```python
from build123d import *

# Parameters (mm, degrees)
BOSS_EXTRUDE1_DEPTH = 3.2
SKETCH3_R           = 12.3
BOSS_EXTRUDE2_DEPTH = 3.2
SKETCH4_R           = 4
BOSS_EXTRUDE3_DEPTH = 4
SKETCH6_W           = 3.2
SKETCH6_H           = 65
BOSS_EXTRUDE4_DEPTH = 190
SKETCH8_W           = 3.2
SKETCH8_H           = 89
BOSS_EXTRUDE5_DEPTH = 190
SKETCH9_W           = 194.2
SKETCH9_H           = 190
BOSS_EXTRUDE7_DEPTH = 3.2


with BuildPart() as part:
    # Sketch1 → Boss-Extrude1 (new body)
    with BuildSketch(Plane(origin=(0, 0, 0), x_dir=(1, 0, 0), z_dir=(0, 1, 0))):
        Polygon((-71.199297972, 0), (119.800702028, 0), (119.800702028, -90), (46.272924854, -150.155348756), (-15.035731115, -153.181069815), (-74.399297972, -109), (-74.399297972, -65), (-71.199297972, -65), align=None)
    boss_extrude1 = extrude(amount=BOSS_EXTRUDE1_DEPTH)

    # Sketch3 → Boss-Extrude2 (add)
    with BuildSketch(Plane.XZ):
        with Locations(Location((-5.399297972, 108.199281837, 0), (0, 0, 270))):
            Circle(SKETCH3_R)
    extrude(amount=BOSS_EXTRUDE2_DEPTH)

    # Sketch4 → Boss-Extrude3 (add)
    with BuildSketch(Plane.XZ.offset(3.2)):
        with Locations(Location((-5.399297972, 108.199281837, 0), (0, 0, 270))):
            Circle(SKETCH4_R)
    extrude(amount=BOSS_EXTRUDE3_DEPTH)

    # Sketch6 → Boss-Extrude4 (add)
    with BuildSketch(Plane(origin=(0, 0, 0), x_dir=(1, 0, 0), z_dir=(0, 1, 0))):
        with Locations((-72.799297972, -32.5)):
            Rectangle(SKETCH6_W, SKETCH6_H)
    extrude(amount=BOSS_EXTRUDE4_DEPTH)

    # Sketch8 → Boss-Extrude5 (add)
    with BuildSketch(Plane(origin=(0, 0, 0), x_dir=(1, 0, 0), z_dir=(0, 1, 0))):
        with Locations((118.200702028, -44.5)):
            Rectangle(SKETCH8_W, SKETCH8_H)
    extrude(amount=BOSS_EXTRUDE5_DEPTH)

    # Mirror1: Boss-Extrude1 across plane
    add(boss_extrude1.mirror(Plane(origin=(0, 95, 0), x_dir=(0, 0, 1), z_dir=(0, -1, 0))))

    # Sketch9 → Boss-Extrude7 (add)
    with BuildSketch(Plane.XY):
        with Locations((22.700702028, 95)):
            Rectangle(SKETCH9_W, SKETCH9_H)
    extrude(amount=-BOSS_EXTRUDE7_DEPTH)


solid = part.part
```
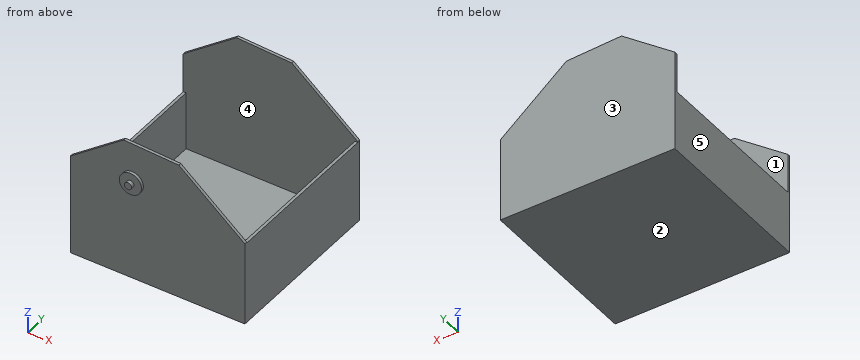
Design review of the part built by this model. Coordinates are the model's own, in mm. Face numbers are marked on the shaded views. A direction names the side the tool comes from. Give positions to 0.01 mm unless a question says otherwise; leave off trailing zeros. Write each loop counter-clockwise with the first axis right and the second up, starting at its lowest first coordinate (ties: lowest second). Pieces come first, ordered by that corner, then holes. Notation, with made-up numbers: (-29.75, 6) -> (-14.75, 6) arc R25 ccw to (-14.75, 27) -> close; hole circle Ø3 at (30.5, -2). An arc over 180 degrees is marked (long way). Answer in a Markdown table with one row per item.
(1) For the marked faces 1 and 2, list the 3-axis set-ups (+Z, -Z, +X, -X, +Y, -Y) from which the entire face can be reached by the end or side of a thin tool; tool diameter is ignored.
Results:
| item | result |
|---|---|
| face 1 | +Z |
| face 2 | -Z, +X, -X, +Y, -Y |
(2) To check wall thickness, follow probe 1 along X at (y, z) = (65, 45.5); probe 2 along Y at (x, z) = (-28, 65); probe 3 along Z at (x, y) = (-21.5, 139.5). State the ranges of each line that lie inside material, in increasing order.
Results:
| item | result |
|---|---|
| probe 1 | -74.4 to -71.2, 116.6 to 119.8 |
| probe 2 | 0 to 3.2, 186.8 to 190 |
| probe 3 | -3.2 to 0 |
(3) Mouldability with a two-part tool opening along X and no side actions: class the marked faces 3, 4 and 5 as +X half, -X half, draft (parallel to the pull), parting line (faces both ways), or undercut.
Results:
| item | result |
|---|---|
| face 3 | draft |
| face 4 | undercut |
| face 5 | -X half |
(4) Consider section C-C (z = 135.5). State the section outline as (x, y) points.
Results:
| item | result |
|---|---|
| outline | (-38.79, 0) -> (64.19, 0) -> (64.19, 3.2) -> (-38.79, 3.2) -> close; (-38.79, 186.8) -> (64.19, 186.8) -> (64.19, 190) -> (-38.79, 190) -> close |
(5) Consider section D-D (x = 36). State the section outline as (y, z) points, then the cut area to 3 significant figures.
Results:
| item | result |
|---|---|
| outline | (0, -3.2) -> (190, -3.2) -> (190, 150.66) -> (186.8, 150.66) -> (186.8, 0) -> (3.2, 0) -> (3.2, 150.66) -> (0, 150.66) -> close |
| area | 1,570 mm2 |
(6) Consider section A-A (z = 10.5). State the section outline as (x, y) points, then the cut area to 3 significant figures.
Results:
| item | result |
|---|---|
| outline | (-74.4, 0) -> (119.8, 0) -> (119.8, 190) -> (-74.4, 190) -> close; hole (-71.2, 3.2) -> (116.6, 3.2) -> (116.6, 186.8) -> (-71.2, 186.8) -> close |
| area | 2,420 mm2 |
(7) Consider section B-B (y = 40.5). State the section outline as (x, z) points, then the cut area to 3 significant figures.
Results:
| item | result |
|---|---|
| outline | (-74.4, -3.2) -> (119.8, -3.2) -> (119.8, 89) -> (116.6, 89) -> (116.6, 0) -> (-71.2, 0) -> (-71.2, 65) -> (-74.4, 65) -> close |
| area | 1,110 mm2 |
(8) Clearance check with flat-ended pins moving along their axes: pin 1 (1.6 mm diameter, centred on x = -73, y = 68, fed in from +Z); pin 2 (6 mm diameter, centred on x = 56.5, z = 64, fed in from -Y); pin 3 (4 mm diameter, centred on x = 2, y = 163.5, fed in from +Z). State where each tip first meets the part, or that it passes through.
Results:
| item | result |
|---|---|
| pin 1 | z = 65 |
| pin 2 | y = 0 |
| pin 3 | z = 0 |
